from build123d import *

# Parameters (mm, degrees)
F1_DEPTH = 2
F0_R     = 1.25
F2_DEPTH = 5.5
F3_R     = 1.99999


# Not quite as in the source:
# - a fillet or chamfer is up to 0.001 mm smaller than in the source, because OpenCascade refuses the exact size
# - a feature names something its author has since deleted; it is built from what else it names


with BuildPart() as f1:
    # F0 (on Top) → F1 (new body)
    with BuildSketch(Plane.XY):
        Polygon((-2, 6.1276243068), (-2, -6.1276243068), (2, -7), (2, 7), align=None)
    extrude(amount=F1_DEPTH)

    # F0 (on Top) → F2 (join)
    with BuildSketch(Plane.XY):
        Polygon((-2, 11.5), (-2, 6.1276243068), (2, 7), (2, 11.5), align=None)
        with Locations((0, 8.5)):
            Circle(F0_R, mode=Mode.SUBTRACT)
        Polygon((-2, -11.5), (2, -11.5), (2, -8.2029914483), (2, -7), (-2, -6.1276243068), align=None)
        with Locations((0, -8.5)):
            Circle(F0_R, mode=Mode.SUBTRACT)
    extrude(amount=F2_DEPTH)

    # F3 (radius 2 in the source; OpenCascade refuses exactly that, so slightly less here)
    f3_edges = [f1.edges().sort_by_distance(p)[0] for p in [
        (2, 11.5, 2.75),
        (-2, 11.5, 2.75),
        (2, -11.5, 2.75),
        (-2, -11.5, 2.75),
        (2, -7, 3.75),
        (2, 7, 3.75),
    ]]
    fillet(f3_edges, radius=F3_R)


solid = f1.part
Read the model definition and answer for the solid it produces. Units are mm, in the model's axes. A direction names the side the tool comes from. Round coordinates to 2 decimals unless told otherwise and drop trailing zeros. Loops run counter-clockwise (first coordinate to the right, second up) from the corner with the lowest first, then second, coordinate; pieces in that order, holes last.
Q1. Section B-B on x = -0.5 is taken. Write down the section's boundary in (y, z), and give its area (3 significant figures).
Q2. Determine the mould class of faces 1 (the face through (-1.43, 10.9, 2.79)), 2 (the face through (2, 0, 1.5)), 3 (the face through (-0.27, -9.72, 2.71)) for opening direction X: released by +X, released by -X, zero draft, split by the parting line, or undercut.
Q3. Which of the six approach directions +Z, -Z, +X, -X, +Y, -Y give full straight-line access (tool end or side, diameter ignored) to faces 4 (the face through (-0.77, -6.396, 3.726)), 5 (the face through (0, 0, 0))?
Q4. Each of these flat-tipped pins is pushed along its axis until it touches: pin 1 (1 mm diameter, centred on y = -3.5, z = 3.5, fed in from +X); pin 2 (2 mm diameter, centred on x = 1, y = -4, fed in from +Z). Where does it stop, or does it pass through?
Q5. Section D-D on y = 3 is taken. Write down the section's boundary in (x, z), and give its area (3 significant figures).
Q6. Section C-C on x = -1.65 is taken. Write down the section's boundary in (y, z).
Q7. Section A-A on z = 2.25 is taken. Give the number of separate pieces and of enclosed holes in the cut face, and give its area (3 significant figures).
Q8. Consider probe 1 along Y at (x, z) = (0, 1.2); probe 2 along Y at (x, z) = (0, 3.15); probe 3 along Y at (x, z) = (-0.8, 3.2). Determine where each line is inside the solid, lowest interval first.
Output:
1. outline: (-11.44, 0) - (-9.65, 0) - (-9.65, 5.5) - (-11.44, 5.5) - close; (-7.35, 0) - (7.35, 0) - (7.35, 5.5) - (6.45, 5.5) - (6.45, 2) - (-6.45, 2) - (-6.45, 5.5) - (-7.35, 5.5) - close; (9.65, 0) - (11.44, 0) - (11.44, 5.5) - (9.65, 5.5) - close
1. area: 55.4 mm2
2. face 1: released by -X
2. face 2: released by +X
2. face 3: undercut
3. face 4: +Z, +X
3. face 5: -Z, +X, -X, +Y, -Y
4. pin 1: passes through
4. pin 2: stops at z = 2
5. outline: (-2, 0) - (2, 0) - (2, 2) - (-2, 2) - close
5. area: 8.00 mm2
6. outline: (-10.63, 0) - (10.63, 0) - (10.63, 5.5) - (6.2, 5.5) - (6.2, 2) - (-6.2, 2) - (-6.2, 5.5) - (-10.63, 5.5) - close
7. separate pieces: 2
7. enclosed holes: 2
7. area: 25.2 mm2
8. probe 1: y = -11.5 to -9.75, -7.25 to 7.25, 9.75 to 11.5
8. probe 2: y = -11.5 to -9.75, -7.25 to -6.56, 6.56 to 7.25, 9.75 to 11.5
8. probe 3: y = -11.33 to -9.46, -7.54 to -6.39, 6.39 to 7.54, 9.46 to 11.33
